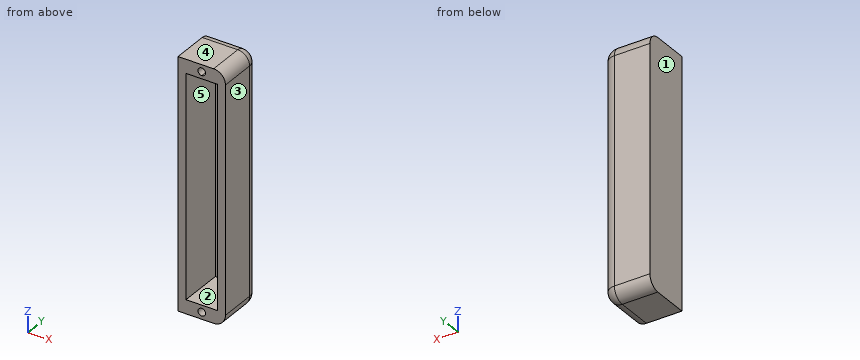
from build123d import *

# Parameters (mm, degrees)
F0_W     = 24
F0_H     = 126
F0_W_2   = 16
F0_H_2   = 112
F1_DEPTH = 24.5
F2_DEPTH = 2
F3_R     = 1.9
F4_DEPTH = 7
F5_R     = 6


with BuildPart() as f1:
    # F0 (on Front) → F1 (new body)
    with BuildSketch(Plane.XZ):
        Rectangle(F0_W, F0_H)
        Rectangle(F0_W_2, F0_H_2, mode=Mode.SUBTRACT)
    extrude(amount=F1_DEPTH)

    # F0 (on Front) → F2 (join)
    with BuildSketch(Plane.XZ):
        Rectangle(F0_W_2, F0_H_2)
    extrude(amount=F2_DEPTH)

    # F3 (on face) → F4 (cut)
    with BuildSketch(Plane.XZ.offset(24.5)):
        with BuildLine():
            ThreePointArc((0, 57.6), (1.343503, 58.156497), (1.9, 59.5))
            ThreePointArc((1.9, 59.5), (1.343503, 60.843503), (0, 61.4))
            Line((0, 61.4), (0, 57.6))
        make_face()
        with BuildLine():
            Line((0, 57.6), (0, 61.4))
            ThreePointArc((0, 61.4), (-1.9, 59.5), (0, 57.6))
        make_face()
        with Locations((0, -59.5)):
            Circle(F3_R)
    extrude(amount=-F4_DEPTH, mode=Mode.SUBTRACT)

    # F5
    f5_edges = [f1.edges().sort_by_distance(p)[0] for p in [
        (0, 0, 63),
        (12, 0, 0),
        (0, 0, -63),
        (12, -12.25, -63),
        (12, -12.25, 63),
    ]]
    fillet(f5_edges, radius=F5_R)


solid = f1.part
Can you work these out from the model? Positions are in its coordinate system, mm. Face numbers are marked on the shaded views. A direction names the side the tool comes from. Coordinates: 2 decimals unless noted, no trailing zeros. Loops run counter-clockwise (first coordinate to the right, second up) from the corner with the lowest first, then second, coordinate; pieces in that order, holes last. Notation, with made-up numbers: (22.5, 4) - (57.5, 4) arc R9 cw to (57.5, 10) - close; hole circle Ø3 at (25.5, 42.25). An arc over 180 degrees is marked (long way). Answer as a JSON object with one key per item and string values. Group by question number.
Item 1: If we section it at B-B (y = -9.75): List the corners of the cut face in (x, z) for me.
Item 2: If we section it at A-A (y = -22.25): List the corners of the cut face in (x, z) for me, plus the area to 3 significant figures.
Item 3: If we mould it in two halves opening along Z, with no side actions, what happens to the marked faces 3, 4 and 5? For each: released by +Z, released by -Z, zero draft, split by the parting line, or undercut.
Item 4: If we section it at C-C (z = -36): List the corners of the cut face in (x, y) for me.
Item 5: On a 3-axis mill with a long thin cutter (end or side, diameter ignored), from which of +Z, -Z, +X, -X, +Y, -Y can I reach the whole of each face in a straight line? I mean the marked faces 1 and 2. Say none if no direction works.
Item 6: If I drill on L1, parallel to X at y = -16.5, z = 52; L2, parallel to Z at x = 1.5, y = -6.5; L3, parallel to Y at x = -1.75, z = -23, over which ranges is the centre line in solid material (lowest first)? Write a range as from..to.
Item 7: For pin 1 (1.5 mm diameter, centred on x = 5.5, y = -5, fed in from +Z); pin 2 (1.5 mm diameter, centred on x = -3, z = 49, fed in from -Y); pin 3 (3 mm diameter, centred on x = 0, z = -59.5, fed in from +Y), each with a flat end and sliding along its axis, tell me the tip position at first contact or that it passes through.
Item 8: If we section it at D-D (x = -6): List the corners of the cut face in (y, z) for me, plus the area to 3 significant figures.
Returned:
{
 "1": {"outline": "(-12, -63) - (6, -63) arc R6 ccw to (12, -57) - (12, 57) arc R6 ccw to (6, 63) - (-12, 63) - close; hole (-8, -56) - (8, -56) - (8, 56) - (-8, 56) - close"},
 "2": {"outline": "(-12, -63) - (6, -63) arc R6 ccw to (12, -57) - (12, 57) arc R6 ccw to (6, 63) - (-12, 63) - close; hole (-8, -56) - (8, -56) - (8, 56) - (-8, 56) - close; hole circle Ø3.8 at (0, -59.5); hole circle Ø3.8 at (0, 59.5)", "area": "1,190 mm²"},
 "3": {"face 3": "zero draft", "face 4": "released by +Z", "face 5": "undercut"},
 "4": {"outline": "(-12, -24.5) - (-8, -24.5) - (-8, -2) - (8, -2) - (8, -24.5) - (12, -24.5) - (12, -6) arc R6 ccw to (6, 0) - (-12, 0) - close"},
 "5": {"face 1": "+Z, -Z, -X, +Y, -Y", "face 2": "-Y"},
 "6": {"L1": "x = -12..-8, 8..12", "L2": "z = -63..-56, 56..63", "L3": "y = -2..0"},
 "7": {"pin 1": "stops at z = 62.99", "pin 2": "stops at y = -2", "pin 3": "stops at y = -0.08"},
 "8": {"outline": "(-24.5, -63) - (-6, -63) arc R6 ccw to (0, -57) - (0, 57) arc R6 ccw to (-6, 63) - (-24.5, 63) - (-24.5, 56) - (-2, 56) - (-2, -56) - (-24.5, -56) - close", "area": "552 mm²"}
}
